Geometry check sheet. Reference: the model listing, model coordinates, mm. A direction names the side the tool comes from. Coordinates: 2 decimals unless noted, no trailing zeros. Write each loop counter-clockwise with the first axis right and the second up, starting at its lowest first coordinate (ties: lowest second). Pieces come first, ordered by that corner, then holes. Notation, with made-up numbers: (7.5, -20.75) -> (28.5, -20.75) arc R24 ccw to (28.5, 7.25) -> close; hole circle Ø3 at (21.25, 80). An arc over 180 degrees is marked (long way). Answer in a Markdown table with one row per item. Add a question column.
Q1. Section check A-A, the plane x = -5. Record the boundary of the cut face in (y, z) (3 decimals), and give its area (3 significant figures).
Q2. Thickness scan on line 1 (X direction, y = 4.5, z = 0); line 2 (Y direction, x = 5.75, z = -4.25) (3 decimals); line 3 (Z direction, x = 1.5, y = 2.5). Record the ranges inside material, lowest first.
Q3. Section check B-B, the plane z = 1.27. Record the boundary of the cut face in (x, y) (3 decimals), and give its area (4 significant figures).
Q4. Section check C-C, the plane y = 0.2. Record the boundary of the cut face in (x, z), and give its area (3 significant figures).
Q5. Tool access check on faces 1 (the face through (-1, 3, -2)), 2 (the face through (4, 3, -2)), 3 (the face through (1, 3, 0.29)). Record the directions out of +Z, -Z, +X, -X, +Y, -Y that give a thin tool (end or side, any length) a straight path to the whole face; none if there is none.
Q6. Gauge pin test, flat ends, axial feed: P1, Ø3, axis at y = 3, z = -2, coming from the +X side; P2, Ø2, axis at x = 8.5, z = 0, coming from the +Y side (3 decimals); P3, Ø1.5, axis at y = 2.5, z = 1.5, coming from the -X side; P4, Ø1.2, axis at y = 2, z = -3, coming from the -X side. Record the tip position at first contact, or that the pin passes through.
Q7. Section check D-D, the plane z = -3.81. Record the boundary of the cut face in (x, y) (3 decimals), and give its area (3 significant figures).
```python
from build123d import *

# Parameters (mm, degrees)
SKETCH1_R           = 1.25
SKETCH1_R_2         = 0.5
BOSS_EXTRUDE1_DEPTH = 0.875
SKETCH2_W           = 5
SKETCH2_H           = 5
BOSS_EXTRUDE2_DEPTH = 4


with BuildPart() as part:
    # Sketch1 → Boss-Extrude1 (new, symmetric)
    with BuildSketch(Plane(origin=(0, 0, 0), x_dir=(1, 0, 0), z_dir=(0, 1, 0))):
        with BuildLine():
            Line((-7.5, 5.71), (7.5, 5.71))
            ThreePointArc((7.5, 5.71), (9.621320344, 4.831320344), (10.5, 2.71))
            Line((10.5, 2.71), (10.5, -2.71))
            ThreePointArc((10.5, -2.71), (9.621320344, -4.831320344), (7.5, -5.71))
            Line((7.5, -5.71), (-7.5, -5.71))
            Line((-7.5, -5.71), (-7.5, 5.71))
        make_face()
        with Locations(Location((7.75, 3.29, 0), (0, 0, 270))):
            Circle(SKETCH1_R, mode=Mode.SUBTRACT)
        with Locations(Location((-5, 3.81, 0), (0, 0, 270))):
            Circle(SKETCH1_R_2, mode=Mode.SUBTRACT)
        with Locations(Location((-5, 1.27, 0), (0, 0, 270))):
            Circle(SKETCH1_R_2, mode=Mode.SUBTRACT)
        with Locations(Location((-5, -1.27, 0), (0, 0, 270))):
            Circle(SKETCH1_R_2, mode=Mode.SUBTRACT)
        with Locations(Location((-5, -3.81, 0), (0, 0, 270))):
            Circle(SKETCH1_R_2, mode=Mode.SUBTRACT)
    extrude(amount=BOSS_EXTRUDE1_DEPTH, both=True)

    # Sketch2 → Boss-Extrude2 (add)
    with BuildSketch(Plane(origin=(0, 0.875, 0), x_dir=(1, 0, 0), z_dir=(0, 1, 0))):
        with Locations((1.5, 2.21)):
            Rectangle(SKETCH2_W, SKETCH2_H)
    extrude(amount=BOSS_EXTRUDE2_DEPTH)


solid = part.part
```
Calculated:
| question | item | result |
|---|---|---|
| 1 | outline | (-0.875, -5.71) -> (0.875, -5.71) -> (0.875, -4.31) -> (-0.875, -4.31) -> close; (-0.875, -3.31) -> (0.875, -3.31) -> (0.875, -1.77) -> (-0.875, -1.77) -> close; (-0.875, -0.77) -> (0.875, -0.77) -> (0.875, 0.77) -> (-0.875, 0.77) -> close; (-0.875, 1.77) -> (0.875, 1.77) -> (0.875, 3.31) -> (-0.875, 3.31) -> close; (-0.875, 4.31) -> (0.875, 4.31) -> (0.875, 5.71) -> (-0.875, 5.71) -> close |
| 1 | area | 13.0 mm² |
| 2 | line 1 | x = -1 to 4 |
| 2 | line 2 | y = -0.875 to 0.875 |
| 2 | line 3 | z = -4.71 to 0.29 |
| 3 | outline | (-7.5, -0.875) -> (-5.5, -0.875) -> (-5.5, 0.875) -> (-7.5, 0.875) -> close; (-4.5, -0.875) -> (10.5, -0.875) -> (10.5, 0.875) -> (-4.5, 0.875) -> close |
| 3 | area | 29.75 mm² |
| 4 | outline | (-7.5, -5.71) -> (7.5, -5.71) arc R3 ccw to (10.5, -2.71) -> (10.5, 2.71) arc R3 ccw to (7.5, 5.71) -> (-7.5, 5.71) -> close; hole circle Ø1 at (-5, -3.81); hole circle Ø1 at (-5, -1.27); hole circle Ø1 at (-5, 1.27); hole circle Ø1 at (-5, 3.81); hole circle Ø2.5 at (7.75, -3.29) |
| 4 | area | 194 mm² |
| 5 | face 1 | +Z, -Z, -X, +Y |
| 5 | face 2 | +Z, -Z, +X, +Y |
| 5 | face 3 | +Z, +X, -X, +Y |
| 6 | P1 | stops at x = 4 |
| 6 | P2 | stops at y = 0.875 |
| 6 | P3 | passes through |
| 6 | P4 | stops at x = -1 |
| 7 | outline | (-7.5, -0.875) -> (-5.5, -0.875) -> (-5.5, 0.875) -> (-7.5, 0.875) -> close; (-4.5, -0.875) -> (6.613, -0.875) -> (6.613, 0.875) -> (4, 0.875) -> (4, 4.875) -> (-1, 4.875) -> (-1, 0.875) -> (-4.5, 0.875) -> close; (8.887, -0.875) -> (10.291, -0.875) -> (10.291, 0.875) -> (8.887, 0.875) -> close |
| 7 | area | 45.4 mm² |
